```python
from build123d import *

# Parameters (mm, degrees)
BOSS_EXTRUDE1_DEPTH     = 3.175
CUT_EXTRUDE1_DEPTH      = 15.674509254
CUT_EXTRUDE1_DEPTH_BACK = 15.674509254
CUT_EXTRUDE2_DEPTH      = 15.674509254


with BuildPart() as part:
    # Sketch1 → Boss-Extrude1 (new, symmetric)
    with BuildSketch(Plane.XY):
        Polygon((5.207, 0), (-5.207, 0), (-5.207, 13.3472), (-3.429, 13.3472), (-3.429, 1.778), (3.429, 1.778), (3.429, 13.3472), (5.207, 13.3472), align=None)
    extrude(amount=BOSS_EXTRUDE1_DEPTH, both=True)

    # Sketch2 → Cut-Extrude1 (cut, two sides: drawn at the far end of the back side and taken through both)
    with BuildSketch(Plane(origin=(0, 0, 0), x_dir=(0, 0, -1), z_dir=(1, 0, 0)).offset(-CUT_EXTRUDE1_DEPTH_BACK)):
        with BuildLine():
            Line((1.4732, 13.3472), (1.4732, 11.874))
            ThreePointArc((1.4732, 11.874), (0, 10.4008), (-1.4732, 11.874))
            Line((-1.4732, 11.874), (-1.4732, 13.3472))
            ThreePointArc((-1.4732, 13.3472), (0, 14.8204), (1.4732, 13.3472))
        make_face()
    extrude(amount=CUT_EXTRUDE1_DEPTH + CUT_EXTRUDE1_DEPTH_BACK, mode=Mode.SUBTRACT)

    # Sketch4 → Cut-Extrude2 (cut, symmetric)
    with BuildSketch(Plane(origin=(0, 0, 0), x_dir=(0, 0, -1), z_dir=(1, 0, 0))):
        Polygon((-3.175, 1.778), (-3.175, 13.3472), (-2.54, 13.3472), align=None)
    cut_extrude2 = extrude(amount=CUT_EXTRUDE2_DEPTH, both=True, mode=Mode.SUBTRACT)

    # Mirror1: Cut-Extrude2 across plane
    add(cut_extrude2.mirror(Plane.XY), mode=Mode.SUBTRACT)

    # Sketch3 → Cut-Revolve1 (revolve, cut)
    with BuildSketch(Plane.XY):
        with BuildLine():
            Line((-3.11999347, 1.905), (3.11999347, 1.905))
            ThreePointArc((3.11999347, 1.905), (0, 0.6345), (-3.11999347, 1.905))
        make_face()
    revolve(axis=Axis((0, 11.874, 0), (1, 0, 0)), mode=Mode.SUBTRACT)


solid = part.part
```
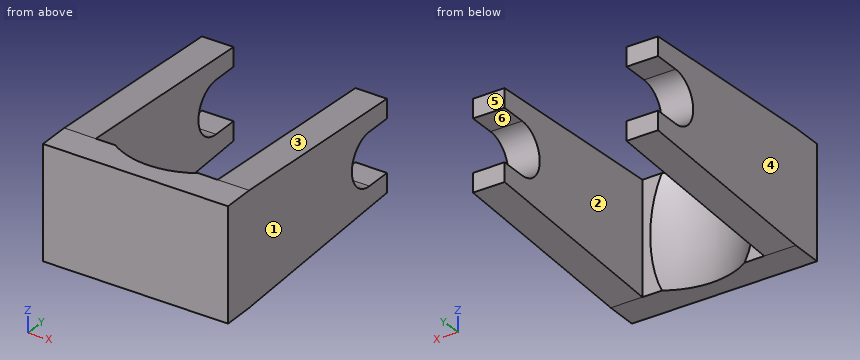
Geometry check sheet. Reference: the model listing, model coordinates, mm. Face numbers are marked on the shaded views. A direction names the side the tool comes from. Coordinates: 2 decimals unless noted, no trailing zeros. Write each loop counter-clockwise with the first axis right and the second up, starting at its lowest first coordinate (ties: lowest second). Pieces come first, ordered by that corner, then holes. Notation, with made-up numbers: M 73,54.25 L 86,54.25 A29 ccw 86,79.25 Z; hole C 56.25,54 d6. An arc over 180 degrees is marked long. Answer as a JSON object with one key per item and string values.
1. Section check C-C, the plane z = 0. Enter the section's corners in (x, y), plus the area to 3 significant figures.
Answers below:
{"outline": "M -5.21,0 L 5.21,0 L 5.21,10.4 L 3.43,10.4 L 3.43,1.78 L 2.98,1.78 A4.47 cw -2.98,1.78 L -3.43,1.78 L -3.43,10.4 L -5.21,10.4 Z", "area": "44.5 mm²"}
2. Draft check along X on the marked faces 1, 2, 3 and 4. Enter one of: released by +X, released by -X, zero draft, split by the parting line, or undercut.
Answers below:
{"face 1": "released by +X", "face 2": "undercut", "face 3": "zero draft", "face 4": "released by -X"}
3. Scan lines: L1, parallel to X at y = 12.75, z = 2.5; L2, parallel to Y at x = -3, z = 0.75; L3, parallel to X at y = 1.25, z = -0.5. Record each from-to range of solid material in increasing order.
Answers below:
{"L1": "x = -5.21 to -3.43, 3.43 to 5.21", "L2": "y = 0 to 1.78", "L3": "x = -5.21 to -2.24, 2.24 to 5.21"}
4. Section check A-A, the plane y = 11.25. Enter the section's corners in (x, z), plus the area to 3 significant figures.
Answers below:
{"outline": "M -5.21,-2.66 L -3.43,-2.66 L -3.43,-1.33 L -5.21,-1.33 Z; M -5.21,1.33 L -3.43,1.33 L -3.43,2.66 L -5.21,2.66 Z; M 3.43,-2.66 L 5.21,-2.66 L 5.21,-1.33 L 3.43,-1.33 Z; M 3.43,1.33 L 5.21,1.33 L 5.21,2.66 L 3.43,2.66 Z", "area": "9.39 mm²"}
5. Section check D-D, the plane y = 3. Enter the section's corners in (x, z).
Answers below:
{"outline": "M -5.21,-3.11 L -3.43,-3.11 L -3.43,3.11 L -5.21,3.11 Z; M 3.43,-3.11 L 5.21,-3.11 L 5.21,3.11 L 3.43,3.11 Z"}
6. Section check B-B, the plane x = 4.25. Enter the section's corners in (y, z) (3 decimals).
Answers below:
{"outline": "M 0,-3.175 L 1.778,-3.175 L 13.347,-2.54 L 13.347,-1.473 L 11.874,-1.473 A1.473 cw 11.874,1.473 L 13.347,1.473 L 13.347,2.54 L 1.778,3.175 L 0,3.175 Z"}
7. Tool access check on the marked faces 5 and 6. Record the directions out of +Z, -Z, +X, -X, +Y, -Y that give a thin tool (end or side, any length) a straight path to the whole face; none if there is none.
Answers below:
{"face 5": "+Z, -Z, +X, -X, +Y", "face 6": "+X, -X, +Y"}
8. Go/stop test with flat-tipped pins: pin 1 Ø1.2 at (x, y) = (4.5, 13) entering from +Z; pin 2 Ø0.5 at (x, z) = (-3, 1) entering from +Y; pin 3 Ø1 at (x, z) = (3.5, 0) entering from +Y. Record where each tip stops, or that it passes through.
Answers below:
{"pin 1": "stops at z = 2.59", "pin 2": "stops at y = 1.78", "pin 3": "stops at y = 10.49"}
